Could you check a few things on this drawing? It's one solid part, dimensions in mm from its lowest x, y, z. A direction names the side the tool comes from. Give positions to 0.01 mm unless a question says otherwise; leave off trailing zeros. Write each loop counter-clockwise with the first axis right and the second up, starting at its lowest first coordinate (ties: lowest second). Pieces come first, ordered by that corner, then holes. Notation, with made-up numbers: M 66.25,29.5 L 110.25,29.5 A10 ccw 110.25,42.5 Z; hole C 87,78.5 d3. An arc over 180 degrees is marked long. Answer as CSV lines item,"result". Start each with the question number.
Q1. Suppose I cut it at B-B (x = 25). Write out the boundary of the cut face in (y, z).
Q2. On a 3-axis mill with a long thin cutter (end or side, diameter ignored), from which of +Z, -Z, +X, -X, +Y, -Y can I reach the whole of each face in a straight line? I mean the marked faces 1, 2, 3 and 4. Say none if no direction works.
Q3. Suppose I cut it at A-A (z = 19). Write out the boundary of the cut face in (x, y), then the cut area to 3 significant figures.
Q4. Suppose I cut it at C-C (y = 28.5). Write out the boundary of the cut face in (x, z), then the cut area to 3 significant figures.
Q5. If I drill on line 1 along Y through (x, z) = (11, 53.5); line 2 along X through (y, z) = (31.5, 42); line 3 along X through (y, z) = (19.5, 25.5), over which ranges is the centre line in solid material (lowest first)?
Q6. For pin 1 (15 mm diameter, centred on x = 9, z = 15.5, fed in from -Y); pin 2 (5 mm diameter, centred on y = 37.5, z = 34.5, fed in from +X); pin 3 (10 mm diameter, centred on y = 37, z = 40, fed in from -X), each with a flat end and sliding along its axis, tell me the tip position at first contact or that it passes through.
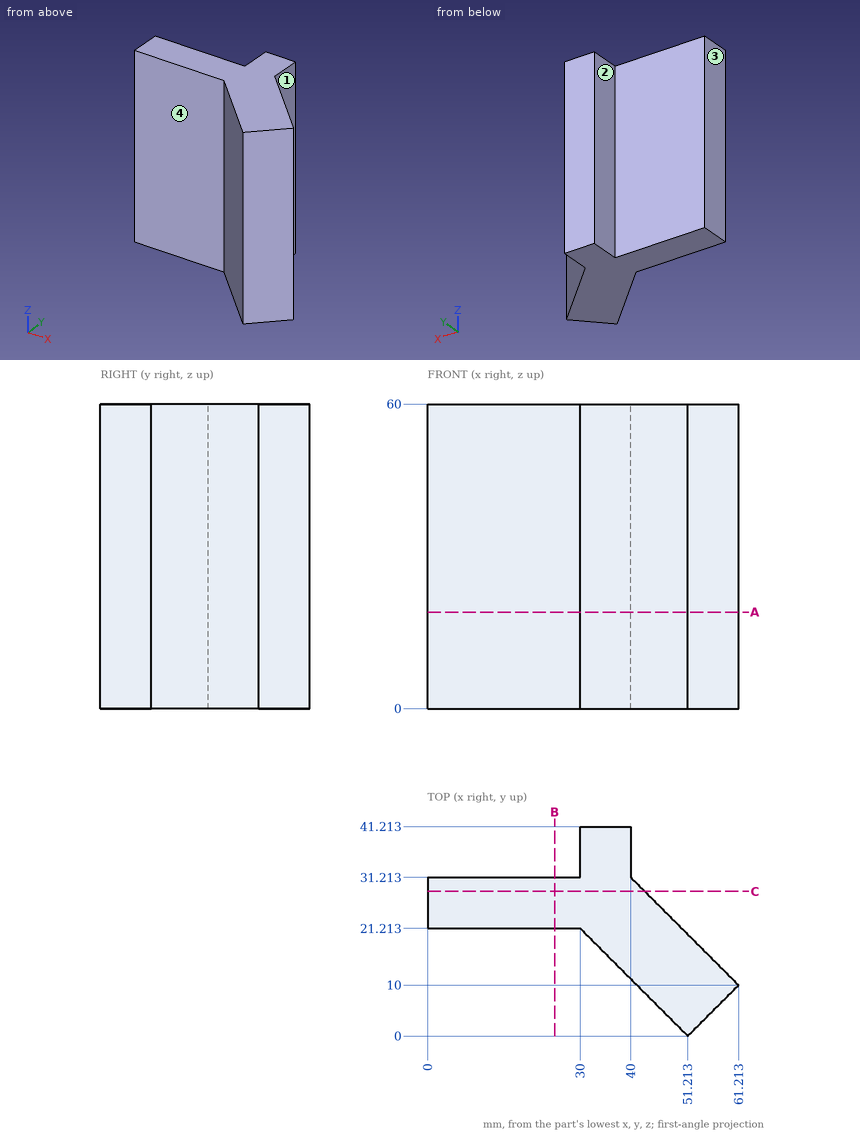
Resolved:
1,outline,"M 21.21,0 L 31.21,0 L 31.21,60 L 21.21,60 Z"
2,face 1,"+Z, -Z, +X, +Y"
2,face 2,"+Z, -Z, -X, +Y"
2,face 3,"+Z, -Z, -X, +Y, -Y"
2,face 4,"+Z, -Z, -X, -Y"
3,outline,"M 0,21.21 L 30,21.21 L 51.21,0 L 61.21,10 L 40,31.21 L 40,41.21 L 30,41.21 L 30,31.21 L 0,31.21 Z"
3,area,"874 mm^2"
4,outline,"M 0,0 L 42.71,0 L 42.71,60 L 0,60 Z"
4,area,"2,560 mm^2"
5,line 1,"21.21 to 31.21"
5,line 2,"30 to 40"
5,line 3,"31.71 to 51.71"
6,pin 1,"y = 21.21"
6,pin 2,"x = 40"
6,pin 3,"x = 30"
